Here's how the part is built. I have some questions about the finished solid (model axes, mm). A direction names the side the tool comes from. Coordinates: 2 decimals unless noted, no trailing zeros. Order: outer loops, then holes, each group sorted by start corner. A loop starts at its lowest first (then second) coordinate and runs counter-clockwise, first axis right, second up. Notation, with made-up numbers: (9, 61) - (46, 61) arc R19 cw to (46, 92) - close; hole circle Ø8 at (-12.5, -28). An arc over 180 degrees is marked (long way). Answer as CSV lines item,"result". Start each with the question number.
Item 1: On a 3-axis mill with a long thin cutter (end or side, diameter ignored), from which of +Z, -Z, +X, -X, +Y, -Y can I reach the whole of each face in a straight line? I mean faces 1 (the face through (117, -78, 10)), 2 (the face through (-4, -2, 11)), 3 (the face through (107.847, -8.749, -37.501)), 4 (the face through (107.995, -9.787, 59.113)). Say none if no direction works.
Item 2: I need wall thicknesses on line 1 (Z direction, x = -68, y = -23.5); line 2 (X direction, y = -57, z = -12.5); line 3 (Y direction, x = -76, z = -9). Which ranges of each line are inside material? Lowest first, please.
Item 3: Imagine slicing it at B-B on x = 5.5. List the corners of the cut face in (y, z) for me, and give its area (3 significant figures).
Item 4: Imagine slicing it at C-C on y = -16.5. List the corners of the cut face in (x, z) for me.
Item 5: We'd pull the mould along Y, two halves only. Please class faces 5 (the face through (27.81, -49.09, 49.31)), 6 (the face through (121.28, -31, 11)), 7 (the face through (22.788, -9.787, -37.587)), 8 (the face through (23.1, -48.67, 47.23)): pulls with the +Y half, pulls with the -Y half, needs draft (parallel to the pull), parting line crosses it, or undercut.
Item 6: I'm going to push flat-ended pins straight in: pin 1 (4 mm diameter, centred on x = 114, y = -79, fed in from -Z); pin 2 (3 mm diameter, centred on y = -49, z = 22, fed in from -X); pin 3 (1.5 mm diameter, centred on x = 5.5, y = -47, fed in from -Z). Where does each tip first touch, or does it pass through?
Item 7: Imagine slicing it at D-D on z = 53. List the corners of the cut face in (x, y) for me.
Item 8: Imagine slicing it at A-A on z = 15. List the corners of the cut face in (x, y) for me, and give its area (3 significant figures).
from build123d import *

# Parameters (mm, degrees)
F1_DEPTH     = 5
F3_DEPTH     = 25
F5_DEPTH     = 2
F7_DEPTH     = 250
F9_DEPTH     = 248
F11_DEPTH    = 110
F13_W        = 5
F13_H        = 5
F14_DEPTH    = 3
F15_T1_DEPTH = 27.9128784748
F16_DEPTH    = 5
F18_D        = 2
F19_R        = 1.49999


# Not quite as in the source:
# - a fillet or chamfer that OpenCascade refuses, or shapes differently, is made with other operations: its cross-section is extruded or revolved along the edge and cut away or added
# - a fillet or chamfer is up to 0.001 mm smaller than in the source, because OpenCascade refuses the exact size


with BuildPart() as f1:
    # F0 (on Front) → F1 (new body)
    with BuildSketch(Plane.XZ):
        Polygon((20.074704662, 60.7631485909), (-126.7197424916, 60.7631485909), (-126.7197424916, 10.7631485909), (-126.7197424916, -39.2368514091), (20.074704662, -39.2368514091), (50.1353926957, -20.9532961249), (78.9564624429, -20.9532961249), (110.8765751123, -39.2368514091), (123.2802575084, -39.2368514091), (123.2802575084, 10.7631485909), (123.2802575084, 60.7631485909), (110.8765751123, 60.7631485909), (78.9564624429, 42.4795933068), (50.1353926957, 42.4795933068), align=None)
    extrude(amount=F1_DEPTH)

    # F2 (on face) → F3 (join)
    with BuildSketch(Plane.XZ.offset(5)):
        Polygon((-126.7197424916, -39.2368514091), (20.074704662, -39.2368514091), (50.1353926957, -20.9532961249), (78.9564624429, -20.9532961249), (110.8765751123, -39.2368514091), (123.2802575084, -39.2368514091), (123.2802575084, 60.7631485909), (110.8765751123, 60.7631485909), (78.9564624429, 42.4795933068), (50.1353926957, 42.4795933068), (20.074704662, 60.7631485909), (-126.7197424916, 60.7631485909), align=None)
        Polygon((49.574933962, -18.9532961249), (19.5142459283, -37.2368514091), (-124.7197424916, -37.2368514091), (-124.7197424916, 58.7631485909), (19.5142459283, 58.7631485909), (49.574933962, 40.4795933068), (79.4886903674, 40.4795933068), (111.4088030368, 58.7631485909), (121.2802575084, 58.7631485909), (121.2802575084, -37.2368514091), (111.4088030368, -37.2368514091), (79.4886903674, -18.9532961249), align=None, mode=Mode.SUBTRACT)
    extrude(amount=F3_DEPTH)

    # F4 (on face) → F5 (join)
    with BuildSketch(Plane.XZ.offset(30)):
        Polygon((110.8765751123, 60.7631485909), (20.074704662, 60.7631485909), (50.1353926957, 42.4795933068), (78.9564624429, 42.4795933068), align=None)
        Polygon((50.1353926957, -20.9532961249), (20.074704662, -39.2368514091), (110.8765751123, -39.2368514091), (78.9564624429, -20.9532961249), align=None)
    extrude(amount=-F5_DEPTH)

    # F6 (on face) → F7 (join)
    with BuildSketch(Plane.YZ.offset(123.2802575084)):
        Polygon((-80, -9.2368514091), (-30, -39.2368514091), (-30, 60.7631485909), (-80, 30.7631485909), align=None)
    extrude(amount=-F7_DEPTH)

    # F8 (on face) → F9 (cut)
    with BuildSketch(Plane(origin=(-126.7197424916, 0, 0), x_dir=(0, -1, 0), z_dir=(-1, 0, 0))):
        Polygon((78, 29.630767833), (29.4460320701, 58.7631485909), (2, 58.7631485909), (2, -37.2368514091), (29.4460320701, -37.2368514091), (78, -8.1044706511), align=None)
    extrude(amount=-F9_DEPTH, mode=Mode.SUBTRACT)

    # F10 (on face) → F11 (cut)
    with BuildSketch(Plane(origin=(0, 0, -39.2368514091), x_dir=(1, 0, 0), z_dir=(0, 0, -1))):
        Polygon((-126.7197424916, 80), (-126.7197424916, 30), (123.2802575084, 80), align=None)
    extrude(amount=-F11_DEPTH, mode=Mode.SUBTRACT)

    # F13 (on face) → F14 (join)
    with BuildSketch(Plane(origin=(-10.6430670189, -53.2153350945, 0), x_dir=(0.9805806757, -0.1961161351, 0), z_dir=(-0.1961161351, -0.9805806757, 0))):
        with Locations((128.8774899908, 4.3955293489)):
            Rectangle(F13_W, F13_H)
    extrude(amount=F14_DEPTH)

    # F15: fillet of radius 5 on 1 edges, made by hand

    # F15_s2 → F15_t1 (cut)
    with BuildSketch(Plane.XY.offset(-9.5609098885)):
        with BuildLine():
            ThreePointArc((118.1831608869, -78.9805806757), (115.9468261093, -80.7598517163), (113.1012273101, -81.0236056685))
            Line((113.1012273101, -81.0236056685), (117.5948124814, -81.9223227028))
            Line((117.5948124814, -81.9223227028), (118.1831608869, -78.9805806757))
        make_face()
    extrude(amount=F15_T1_DEPTH, mode=Mode.SUBTRACT)

    # F16 (add): a face of the model
    f16_faces = [f1.faces().sort_by_distance(p)[0] for p in [
        (112.9860833057, -79.4708710135, 4.3955293489),
    ]]
    extrude(f16_faces, amount=F16_DEPTH)

    # F18 (through all)
    with Locations(Plane.XY.offset(6.8955293489)):
        with Locations((110.5346316165, -78.9805806757)):
            Hole(F18_D / 2)

    # F19 (radius 1.5 in the source; OpenCascade refuses exactly that, so slightly less here)
    f19_edges = [f1.edges().sort_by_distance(p)[0] for p in [
        (108.377354, -77.019419, 4.395529),
        (107.789006, -79.961161, 4.395529),
    ]]
    fillet(f19_edges, radius=F19_R)


solid = f1.part
Responses:
1,face 1,"none"
1,face 2,"-X"
1,face 3,"-Z, +Y"
1,face 4,"+Z, +Y"
2,line 1,"z = -39.24 to -37.24, 58.76 to 60.76"
2,line 2,"x = 121.28 to 123.28"
2,line 3,"y = -2 to 0"
3,outline,"(-56.44, -23.37) - (-30, -39.24) - (0, -39.24) - (0, 60.76) - (-30, 60.76) - (-56.44, 44.9) - (-56.44, 42.56) - (-30, 58.43) - (-30, 58.76) - (-2, 58.76) - (-2, -37.24) - (-30, -37.24) - (-30, -36.9) - (-56.44, -21.04) - close"
3,area,"435 mm^2"
4,outline,"(-126.72, -39.24) - (20.07, -39.24) - (23.36, -37.24) - (-126.72, -37.24) - close; (-126.72, 58.76) - (23.36, 58.76) - (20.07, 60.76) - (-126.72, 60.76) - close; (107.38, -37.24) - (110.88, -39.24) - (123.28, -39.24) - (123.28, 60.76) - (110.88, 60.76) - (107.38, 58.76) - (121.28, 58.76) - (121.28, -37.24) - close"
5,face 5,"pulls with the -Y half"
5,face 6,"undercut"
5,face 7,"needs draft"
5,face 8,"undercut"
6,pin 1,"stops at z = -11.04"
6,pin 2,"stops at x = 121.28"
6,pin 3,"stops at z = -29.49"
7,outline,"(-126.72, -2) - (32.84, -2) - (32.84, 0) - (-126.72, 0) - close; (-81.46, -39.05) - (-62.03, -42.94) - (123.28, -42.94) - (123.28, 0) - (97.32, 0) - (97.32, -2) - (121.28, -2) - (121.28, -39.05) - close"
8,outline,"(-126.72, -2) - (121.28, -2) - (121.28, -78) - (113.28, -78) - (123.28, -80) - (123.28, 0) - (-126.72, 0) - close"
8,area,"662 mm^2"
